```python
from build123d import *

# Parameters (mm, degrees)
REVOLVE1_ANGLE     = 72
CUT_EXTRUDE2_DEPTH = 0.635
CUT_EXTRUDE3_DEPTH = 0.635
CUT_EXTRUDE4_REACH = 151.001


with BuildPart() as part:
    # Sketch1 → Revolve1 (revolve)
    with BuildSketch(Plane.XY):
        with BuildLine():
            Line((0, 0), (0, 50.8))
            Line((0, 50.8), (88.9, 50.8))
            ThreePointArc((88.9, 50.8), (98.376882891, 26.181720723), (101.6, 0))
            Line((101.6, 0), (0, 0))
        make_face()
    revolve(axis=Axis((0, 0, 0), (0, 1, 0)), revolution_arc=REVOLVE1_ANGLE)

    # Sketch3 → Cut-Extrude2 (cut)
    with BuildSketch(Plane(origin=(0, 0, 0), x_dir=(-0.3090169943749449, 0, 0.9510565162951544), z_dir=(-0.9510565162951544, 0, -0.3090169943749449))):
        with BuildLine():
            Line((0, 50.8), (-88.9, 50.8))
            ThreePointArc((-88.9, 50.8), (-98.376882891, 26.181720723), (-101.6, 0))
            Line((-101.6, 0), (0, 0))
            Line((0, 0), (0, 50.8))
        make_face()
    extrude(amount=-CUT_EXTRUDE2_DEPTH, mode=Mode.SUBTRACT)

    # Sketch4 → Cut-Extrude3 (cut)
    with BuildSketch(Plane.XY):
        with BuildLine():
            Line((0.667678512, 50.8), (0.667678512, 0))
            Line((0.667678512, 0), (101.6, 0))
            ThreePointArc((101.6, 0), (98.376882891, 26.181720723), (88.9, 50.8))
            Line((88.9, 50.8), (0.667678512, 50.8))
        make_face()
    extrude(amount=-CUT_EXTRUDE3_DEPTH, mode=Mode.SUBTRACT)

    # Sketch5 → Cut-Extrude4 (cut, up to next)
    with BuildSketch(Plane(origin=(0, 50.8, 0), x_dir=(1, 0, 0), z_dir=(0, 1, 0)), mode=Mode.PRIVATE) as cut_extrude4_sk1:
        Polygon((1.658905685, 0.635), (0.874002519, 0.635), (1.116550937, 1.38148727), align=None)
    cut_extrude4_tool1 = extrude(cut_extrude4_sk1.sketch, amount=-CUT_EXTRUDE4_REACH, mode=Mode.PRIVATE) & part.part
    add(cut_extrude4_tool1.solids().sort_by_distance((1.216486, 50.8, -0.883829))[0], mode=Mode.SUBTRACT)


solid = part.part
```
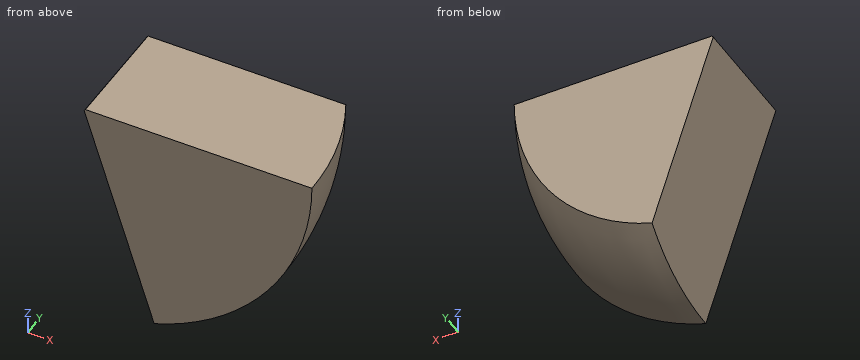
Here's how the part is built. I have some questions about the finished solid (model axes, mm). Coordinates: 2 decimals unless noted, no trailing zeros. Order: outer loops, then holes, each group sorted by start corner. A loop starts at its lowest first (then second) coordinate and runs counter-clockwise, first axis right, second up. Notation, with made-up numbers: M 2,4 L 18,4 A15 cw 18,19 Z; hole C -25.75,19.25 d6. An arc over 180 degrees is marked long. Answer as a JSON object with one key per item and string values. Group by question number.
(1) I need wall thicknesses on probe 1 along X at (y, z) = (25.5, -15); probe 2 along X at (y, z) = (38.5, -76.5); probe 3 along Z at (x, y) = (66, 39) (3 decimals). Which ranges of each line are inside material? Lowest first, please.
(2) Suppose I cut it at A-A, the plane x = 26. Please give me the cut outline in (y, z) (3 decimals).
(3) For pin 1 (2 mm diameter, centred on x = 46.5, y = 31, fed in from -Z); pin 2 (1 mm diameter, centred on x = 39, y = 7, fed in from -Z); pin 3 (5 mm diameter, centred on y = 24, z = -63, fed in from +X), each with a flat end and sliding along its axis, tell me the tip position at first contact or that it passes through.
Values found:
{
 "1": {"probe 1": "x = 5.54 to 97.4", "probe 2": "x = 25.52 to 55.48", "probe 3": "z = -67.366 to -0.635"},
 "2": {"outline": "M 0,-77.965 L 50.8,-77.965 L 50.8,-0.635 L 0,-0.635 Z"},
 "3": {"pin 1": "stops at z = -85.82", "pin 2": "stops at z = -93.78", "pin 3": "stops at x = 78.36"}
}
